Here's the drawing with two shaded views (mm, measured from the low corner). I have some questions. Coordinates: 2 decimals unless noted, no trailing zeros. Write each loop counter-clockwise with the first axis right and the second up, starting at its lowest first coordinate (ties: lowest second). Pieces come first, ordered by that corner, then holes. Notation, with made-up numbers: (-18, 59) -> (29, 59) arc R29 ccw to (29, 79) -> close; hole circle Ø11 at (40, 36). An arc over 180 degrees is marked (long way). Put each result on its own line as item: value. Start each with the question number.
Item 1: I want a section at C-C, the plane x = 16.25. List the corners of the cut face in (y, z) for me, then the cut area to 3 significant figures.
Item 2: I want a section at B-B, the plane y = 5.25. List the corners of the cut face in (x, z) for me, then the cut area to 3 significant figures.
Item 3: I want a section at A-A, the plane z = 1.15. List the corners of the cut face in (x, y) for me, then the cut area to 3 significant figures.
Item 4: I need wall thicknesses on line 1 (X direction, y = 4, z = 0.35); line 2 (X direction, y = 14, z = 0.8); line 3 (Y direction, x = 16.25, z = 1.35). Which ranges of each line are inside material? Lowest first, please. Write a range as [from, to].
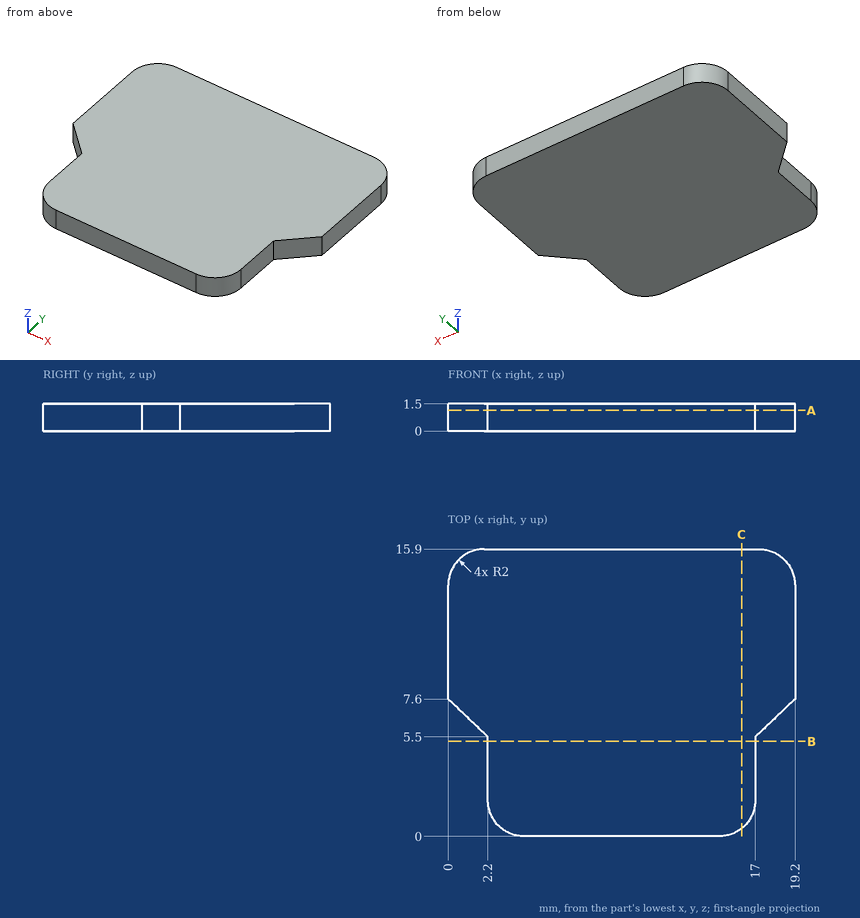
Calculated:
1. outline: (0.44, 0) -> (15.9, 0) -> (15.9, 1.5) -> (0.44, 1.5) -> close
1. area: 23.2 mm2
2. outline: (2.2, 0) -> (17, 0) -> (17, 1.5) -> (2.2, 1.5) -> close
2. area: 22.2 mm2
3. outline: (0, 7.6) -> (2.2, 5.5) -> (2.2, 2) arc R2 ccw to (4.2, 0) -> (15, 0) arc R2 ccw to (17, 2) -> (17, 5.5) -> (19.2, 7.6) -> (19.2, 13.9) arc R2 ccw to (17.2, 15.9) -> (2, 15.9) arc R2 ccw to (0, 13.9) -> close
3. area: 273 mm2
4. line 1: x = [2.2, 17]
4. line 2: x = [0, 19.2]
4. line 3: y = [0.44, 15.9]
